Geometry check sheet. Reference: the model listing, model coordinates, mm. A direction names the side the tool comes from. Coordinates: 2 decimals unless noted, no trailing zeros. Order: outer loops, then holes, each group sorted by start corner. A loop starts at its lowest first (then second) coordinate and runs counter-clockwise, first axis right, second up. Notation, with made-up numbers: (28.25, 12) - (47.25, 12) arc R22 ccw to (47.25, 21) - close; hole circle Ø4 at (24, -32.5). An arc over 180 degrees is marked (long way). Put each result on its own line as item: value.
from build123d import *

# Parameters (mm, degrees)
F0_R     = 6.35
F1_DEPTH = 15.875
F4_R     = 15.875
F4_R_2   = 6.35
F5_DEPTH = 3.175
F6_SIZE  = 0.508


with BuildPart() as f1:
    # F0 (on Top) → F1 (new body)
    with BuildSketch(Plane.XY):
        Polygon((12.7, -7.332348), (12.7, 7.332348), (0, 14.664697), (-12.7, 7.332348), (-12.7, -7.332348), (0, -14.664697), align=None)
        Circle(F0_R, mode=Mode.SUBTRACT)
    extrude(amount=F1_DEPTH)

    # F2 (on Front) → F3 (revolve, cut)
    with BuildSketch(Plane.XZ):
        Polygon((16.705426, 15.875), (12.7, 15.875), (16.705426, 13.562466), align=None)
    revolve(axis=Axis((0, 0, 7.953254), (0, 0, -1)), mode=Mode.SUBTRACT)

    # F4 (on Top) → F5 (join)
    with BuildSketch(Plane.XY):
        Circle(F4_R)
        Circle(F4_R_2, mode=Mode.SUBTRACT)
    extrude(amount=F5_DEPTH)

    # F6
    f6_edges = [f1.edges().sort_by_distance(p)[0] for p in [
        (-6.35, 0, 0),
        (-6.35, 0, 15.875),
    ]]
    chamfer(f6_edges, length=F6_SIZE)


solid = f1.part
Q1. Section check B-B on x = 14. Record the boundary of the cut face in (y, z) (3 decimals).
Answer block:
outline: (-7.484, 0) - (7.484, 0) - (7.484, 3.175) - (-7.484, 3.175) - close
Q2. Draft check along X on faces 5 (the flat face through (7, -3, 0)), 6 (the cylindrical face through (-1.38, -6.2, 7.83)), 7 (the conical face through (-11.4, 6.6, 15.6)). Enter one of: pulls with the +X half, pulls with the -X half, needs draft (parallel to the pull), parting line crosses it, or undercut.
Answer block:
face 5: needs draft
face 6: undercut
face 7: pulls with the -X half
Q3. Access from +Z, -Z, +X, -X, +Y, -Y to the whole of each face (thin tool, end or side, straight path). Record for faces 1 (the flat face through (6.26, -11.05, 9.44)), 2 (the flat face through (6.439, 10.947, 9.436)), 3 (the flat face through (7, 11, 3.175)), 4 (the flat face through (-6.26, 11.05, 9.44)).
Answer block:
face 1: +Z, +X, -Y
face 2: +Z, +X, +Y
face 3: +Z
face 4: +Z, -X, +Y
Q4. Section check A-A on z = 13.5. Record the boundary of the cut face in (x, y), then the cut area to 3 significant figures.
Answer block:
outline: (-12.7, -7.33) - (0, -14.66) - (12.7, -7.33) - (12.7, 7.33) - (0, 14.66) - (-12.7, 7.33) - close; hole circle Ø12.7 at (0, 0)
area: 432 mm^2
Q5. Depth check by flat-ended pin: pin 1 Ø8 at (x, z) = (3.5, 14) entering from -Y; pin 2 Ø7.5 at (x, y) = (0, 0) entering from +Z; pin 3 Ø2 at (x, y) = (3.5, -4.5) entering from -Z; pin 4 Ø5 at (x, z) = (10, 4.5) entering from +Y. Enter the tip coordinate at first touch or a pass-through.
Answer block:
pin 1: stops at y = -14.66
pin 2: passes through
pin 3: stops at z = 0.16
pin 4: stops at y = 13.78
Q6. Thickness scan on L1, parallel to Y at x = 0, z = 8.25; L2, parallel to Z at x = -10, y = 9 (3 decimals); L3, parallel to X at y = 3, z = 9.5. Record the ranges inside material, lowest first. Write a range as [from, to].
Answer block:
L1: y = [-14.66, -6.35], [6.35, 14.66]
L2: z = [0, 3.175]
L3: x = [-12.7, -5.6], [5.6, 12.7]
